```python
from build123d import *

# Parameters (mm, degrees)
F1_DEPTH = 10
F4_R     = 5
F5_R     = 2


with BuildPart() as f1:
    # F0 (on Top) → F1 (new body, symmetric)
    with BuildSketch(Plane.XY):
        Polygon((-22, 0), (0, 0), (0, -20), (3, -20), (3, 10), (-22, 10), align=None)
        with BuildLine():
            Line((3, -20), (0, -20))
            ThreePointArc((0, -20), (1.5, -21.5), (3, -20))
        make_face()
    extrude(amount=F1_DEPTH, both=True)

    # F2 (on Top) → F3 (revolve, cut)
    with BuildSketch(Plane.XY):
        Polygon((-17.0284808531, 5.4523187828), (-16.9238939618, 4.256885145), (3, 6), (7.9809734905, 6.4357787137), (7.8763865992, 7.6312123514), align=None)
    revolve(axis=Axis((-4.4714602357, 5.3463319294, 0), (0.9961946981, 0.0871557427, 0)), mode=Mode.SUBTRACT)

    # F4
    f4_edges = [f1.edges().sort_by_distance(p)[0] for p in [
        (-22, 10, 0),
    ]]
    fillet(f4_edges, radius=F4_R)

    # F5
    f5_edges = [f1.edges().sort_by_distance(p)[0] for p in [
        (3, 10, 0),
        (-22, 0, 0),
    ]]
    fillet(f5_edges, radius=F5_R)


solid = f1.part
```
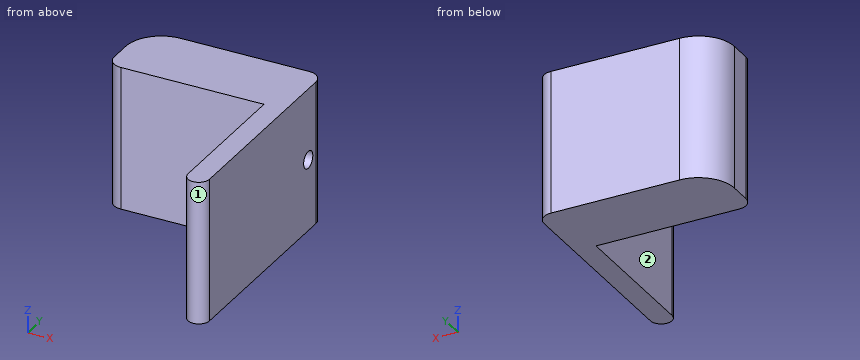
CAD build for the part. Positions are in the model's coordinates, mm. Face numbers are marked on the shaded views. A direction names the side the tool comes from. Round coordinates to 2 decimals unless told otherwise and drop trailing zeros. Write each loop counter-clockwise with the first axis right and the second up, starting at its lowest first coordinate (ties: lowest second). Pieces come first, ordered by that corner, then holes. Notation, with made-up numbers: (-18.75, 16.5) - (-10.75, 16.5) arc R19 ccw to (-10.75, 37.5) - close; hole circle Ø8 at (-12, 59). An arc over 180 degrees is marked (long way). Return JSON: item names as keys, results as strings. Group by question number.
Item 1: Band-saw the part on B-B on y = -8.5. List the corners of the cut face in (x, z).
Item 2: 3-axis set-ups, long thin cutter, end or side, ignore diameter. For the marked faces 1 and 2: which of +Z, -Z, +X, -X, +Y, -Y reach the whole face in a straight line?
Item 3: Band-saw the part on A-A on z = -4.25. List the corners of the cut face in (x, y).
Item 4: Flat gauge pins, fed straight in: pin 1 Ø2 at (x, z) = (-4, 3) entering from -Y; pin 2 Ø10 at (y, z) = (-9, -3.5) entering from -X. Where does each tip first touch, or does it go through?
Item 5: Probe probe 1 along X at (y, z) = (-4, -7.25); probe 2 along Y at (x, z) = (-7.5, -4); probe 3 along X at (y, z) = (5.5, -4). List the from-to ranges inside material, lowest first.
Resolved:
{
 "1": {"outline": "(0, -10) - (3, -10) - (3, 10) - (0, 10) - close"},
 "2": {"face 1": "+Z, -Z, -Y", "face 2": "+Z, -Z, -X, -Y"},
 "3": {"outline": "(-22, 2) arc R2 ccw to (-20, 0) - (0, 0) - (0, -20) arc R1.5 ccw to (3, -20) - (3, 8) arc R2 ccw to (1, 10) - (-17, 10) arc R5 ccw to (-22, 5) - close"},
 "4": {"pin 1": "stops at y = 0", "pin 2": "stops at x = 0"},
 "5": {"probe 1": "x = 0 to 3", "probe 2": "y = 0 to 10", "probe 3": "x = -21.97 to 3"}
}
